```python
from build123d import *

# Parameters (mm, degrees)
SKETCH_1_W          = 260
SKETCH_1_H          = 100
EXTRUDE_1_DEPTH     = 80
SHELL_1_T           = -2
SKETCH_4_W          = 260
SKETCH_4_H          = 70
EXTRUDE_1_2_DEPTH   = 2
CUT_EXTRUDE_3_DEPTH = 10
CHAMFER_1_SIZE      = 50


with BuildPart() as part:
    # 草图1 → Extrude 1 (new body)
    with BuildSketch(Plane.XY):
        with Locations((130, 50)):
            Rectangle(SKETCH_1_W, SKETCH_1_H)
    extrude(amount=EXTRUDE_1_DEPTH)

    # 抽壳1
    shell_1_openings = [part.faces().sort_by_distance(p)[0] for p in [
        (130, 50, 80),
    ]]
    offset(amount=SHELL_1_T, openings=shell_1_openings, kind=Kind.INTERSECTION)

    # 草图4 → Extrude 1 2 (add)
    with BuildSketch(Plane(origin=(0, 100, 0), x_dir=(1, 0, 0), z_dir=(0, 1, 0))):
        with Locations((130, -115)):
            Rectangle(SKETCH_4_W, SKETCH_4_H)
    extrude(amount=-EXTRUDE_1_2_DEPTH)

    # 草图5 → 切除-拉伸3 (cut)
    with BuildSketch(Plane(origin=(0, 98, 0), x_dir=(-1, 0, 0), z_dir=(0, -1, 0))):
        with BuildLine():
            Line((-119, -140), (-119, -134.472135955))
            ThreePointArc((-119, -134.472135955), (-115, -124), (-111, -134.472135955))
            Line((-111, -134.472135955), (-111, -140))
            ThreePointArc((-111, -140), (-115, -144), (-119, -140))
        make_face()
        with BuildLine():
            Line((-149, -140), (-149, -134.472135955))
            ThreePointArc((-149, -134.472135955), (-145, -124), (-141, -134.472135955))
            Line((-141, -134.472135955), (-141, -140))
            ThreePointArc((-141, -140), (-145, -144), (-149, -140))
        make_face()
    extrude(amount=-CUT_EXTRUDE_3_DEPTH, mode=Mode.SUBTRACT)

    # 倒角1
    chamfer_1_edges = [part.edges().sort_by_distance(p)[0] for p in [
        (260, 99, 150),
        (0, 99, 150),
    ]]
    chamfer(chamfer_1_edges, length=CHAMFER_1_SIZE)


solid = part.part
```
Can you work these out from the model? Positions are in its coordinate system, mm. A direction names the side the tool comes from. Give positions to 0.01 mm unless a question says otherwise; leave off trailing zeros. Order: outer loops, then holes, each group sorted by start corner. A loop starts at its lowest first (then second) coordinate and runs counter-clockwise, first axis right, second up. Notation, with made-up numbers: M 11,46 L 48,46 A23 cw 48,67 Z; hole C -6,-31 d7. An arc over 180 degrees is marked long. Write item = value, one per line. Start each with the question number.
Q1. Suppose I cut it at A-A (z = 130). Write out the boundary of the cut face in (x, y).
Q2. For faces 4 (the flat face through (0, 51, 40)), 5 (the flat face through (128, 98, 75)), which set-ups out of +Z, -Z, +X, -X, +Y, -Y let a thin tool reach every point of the face, with its end or its side?
Q3. Suppose I cut it at C-C (y = 21.5). Write out the boundary of the cut face in (x, z).
Q4. Suppose I cut it at B-B (x = 115). Write out the boundary of the cut face in (y, z), plus the area to 3 significant figures.
Q5. I need wall thicknesses on probe 1 along Y at (x, z) = (115, 60); probe 2 along Z at (x, y) = (145, 98.45); probe 3 along X at (y, z) = (99.65, 130). Which ranges of each line are inside material? Lowest first, please. Write a range as [from, to].
Q6. Suppose I cut it at D-D (x = 73). Write out the boundary of the cut face in (y, z).
Q7. We'd pull the mould along Y, two halves only. Please class faces 1 (the flat face through (128, 51, 0)), 2 (the flat face through (128, 0, 39)), 3 (the flat face through (128, 2, 40)): pulls with the +Y half, pulls with the -Y half, needs draft (parallel to the pull), parting line crosses it, or undercut.
Q8. Will these pins go through, and if not, where does the flat tip stop? pin 1 Ø0.6 at (y, z) = (99.5, 138) entering from -X; pin 2 Ø14 at (x, z) = (145, 130) entering from -Y; pin 3 Ø4 at (x, y) = (168, 55) entering from -Z; pin 4 Ø8 at (x, y) = (179.5, 29.5) entering from +Z.
Check result:
q1.outline = M 30,98 L 109,98 L 109,100 L 30,100 Z; M 121,98 L 139,98 L 139,100 L 121,100 Z; M 151,98 L 230,98 L 230,100 L 151,100 Z
q2.face_4 = +Z, -Z, -X, +Y, -Y
q2.face_5 = +Z
q3.outline = M 0,0 L 260,0 L 260,80 L 258,80 L 258,2 L 2,2 L 2,80 L 0,80 Z
q4.outline = M 0,0 L 100,0 L 100,124 L 98,124 L 98,2 L 2,2 L 2,80 L 0,80 Z; M 98,144 L 100,144 L 100,150 L 98,150 Z
q4.area = 612 mm2
q5.probe_1 = [0, 2], [98, 100]
q5.probe_2 = [0, 124], [144, 150]
q5.probe_3 = [30, 109], [121, 139], [151, 230]
q6.outline = M 0,0 L 100,0 L 100,150 L 98,150 L 98,2 L 2,2 L 2,80 L 0,80 Z
q7.face_1 = needs draft
q7.face_2 = pulls with the -Y half
q7.face_3 = undercut
q8.pin_1 = 37.7
q8.pin_2 = 98
q8.pin_3 = 0
q8.pin_4 = 2
